Autodesk Inventor part; units mm, degrees
ref_plane "YZ Plane" through (0, 0, 0) normal (1, 0, 0) x (0, 1, 0)
ref_plane "XZ Plane" through (0, 0, 0) normal (0, 1, 0) x (-1, 0, 0)
ref_plane "XY Plane" through (0, 0, 0) normal (0, 0, 1) x (1, 0, 0)
sketch "Sketch1" plane through (0, 0, 0) normal (0, 1, 0) x (-1, 0, 0)
  line L0 (0, 0) -> (85.48, 0)
  line L1 (85.48, 0) -> (85.48, -127.76)
  line L2 (85.48, -127.76) -> (0, -127.76)
  line L3 (0, -127.76) -> (0, 0)
  line L4 (0, 0) -> (7.0711, -7.0711)
  line L5 (0, 0) -> (10, 0) construction
  circle A0 centre (7.0711, -7.0711) radius 4.7625
  dimension "d0" = 85.48
  dimension "d1" = 127.76
  dimension "offsetDiag" = 10
  dimension "d3" = 45
  dimension "d4" = 9.525
extrude "Extrusion1" add sketch "Sketch1" along normal blind 12.7 contours L0 L1 L2 L3 | A0
sketch "Sketch3" plane through (0, 12.7, 0) normal (0, 1, 0) x (1, 0, 0)
  line L0 (0, 0) -> (0, 127.76)
  line L1 (0, 63.88) -> (-72.5, 63.88)
  line L2 (-140, 121.63) -> (-5, 121.63)
  line L3 (-5, 121.63) -> (-5, 6.13)
  line L4 (-5, 6.13) -> (-140, 6.13)
  line L5 (-140, 6.13) -> (-140, 121.63)
  line L6 (-140, 121.63) -> (-5, 6.13) construction
  line L7 (-5, 121.63) -> (-140, 6.13) construction
  dimension "d23" = 72.5
  dimension "d24" = 135
  dimension "d25" = 115.5
extrude "Extrusion2" cut sketch "Sketch3" against normal blind 2.54
sketch "Sketch4" plane through (0, 12.7, 0) normal (0, 1, 0) x (1, 0, 0)
  line L0 (-5, 121.63) -> (-5, 6.13)
  line L1 (5, 67.055) -> (-5, 67.055)
  line L2 (-5, 67.055) -> (-5, 60.705)
  line L3 (-5, 60.705) -> (5, 60.705)
  line L4 (5, 60.705) -> (5, 67.055)
  line L5 (0, 0) -> (0, 127.76)
  line L6 (5, 67.055) -> (-5, 60.705) construction
  line L7 (-5, 67.055) -> (5, 60.705) construction
  point P0 (0, 63.88)
  point P1 (0, 60.705)
  point P2 (0, 67.055)
  dimension "d28" = 6.35
extrude "Extrusion3" cut sketch "Sketch4" against normal blind 2.54 contours L1 L5 L3 L0
sketch "Sketch5" plane through (0, 12.7, 0) normal (0, 1, 0) x (1, 0, 0)
  line L0 (0, 67.055) -> (0, 60.705)
  line L1 (0, 63.88) -> (-67.5, 63.88)
  circle A0 centre (-67.5, 63.88) radius 13.335
  line L2 (-85.48, 0) -> (0, 0)
  line L3 (-70.04, 127.76) -> (-38.29, 127.76)
  line L4 (-38.29, 127.76) -> (-38.29, 0)
  line L5 (-38.29, 0) -> (-70.04, 0)
  line L6 (-70.04, 0) -> (-70.04, 127.76)
  line L7 (-70.04, 127.76) -> (-38.29, 0) construction
  line L8 (-38.29, 127.76) -> (-70.04, 0) construction
  line L9 (-85.48, 121.63) -> (-5, 121.63)
  line L10 (-68.5166, 121.63) -> (-38.29, 121.63)
  line L11 (-38.29, 121.63) -> (-38.29, 127.76)
  line L12 (-38.29, 127.76) -> (-68.5166, 127.76)
  line L13 (-68.5166, 127.76) -> (-68.5166, 121.63)
  line L14 (-5, 6.13) -> (-85.48, 6.13)
  line L15 (-70.04, 0) -> (-38.29, 0)
  line L16 (-38.29, 0) -> (-38.29, 6.13)
  line L17 (-38.29, 6.13) -> (-70.04, 6.13)
  line L18 (-70.04, 6.13) -> (-70.04, 0)
  circle A1 centre (-67.5, 63.88) radius 14.9695
  point P0 (-54.165, 63.88)
  point P1 (-70.04, 6.13)
  point P2 (-38.29, 121.63)
  dimension "d32" = 26.67
  dimension "d31" = 67.5
  dimension "d33" = 31.75
  dimension "d158" = 29.939
sketch "Sketch22" plane through (0, 12.7, 0) normal (0, 1, 0) x (1, 0, 0)
  line L0 (0, 127.76) -> (-85.48, 127.76)
  line L1 (0, 0) -> (0, 127.76)
  line L2 (-85.48, 127.76) -> (0, 127.76)
  line L3 (0, 127.76) -> (0, 121.1763)
  line L4 (0, 121.1763) -> (-85.48, 121.1763)
  line L5 (-85.48, 121.1763) -> (-85.48, 127.76)
  line L6 (0, 0) -> (0, 60.705)
  line L7 (-5, 6.13) -> (-85.48, 6.13)
  line L8 (0, 0) -> (-85.48, 0)
  line L9 (-85.48, 0) -> (-85.48, 6.13)
  line L10 (-85.48, 6.13) -> (0, 6.13)
  line L11 (0, 6.13) -> (0, 0)
extrude "Extrusion16" add sketch "Sketch22" along normal blind 6.35
sketch "Sketch23" plane through (0, 19.05, 0) normal (0, 1, 0) x (1, 0, 0)
  line L0 (0, 127.76) -> (-85.48, 127.76)
  line L1 (-85.48, 0) -> (0, 0)
  line L2 (-85.48, 127.76) -> (0, 127.76)
  line L3 (0, 127.76) -> (0, 0)
  line L4 (0, 0) -> (-85.48, 0)
  line L5 (-85.48, 0) -> (-85.48, 127.76)
extrude "Extrusion17" add sketch "Sketch23" along normal blind 25.4
extrude "Extrusion18" cut sketch "Sketch5" along normal blind 38.1 contours A1 L6 A0 L1 | L1 A0 L6 A1 | A0 L6 | L6 A0 A1 | L6 A0
pattern_linear "Rectangular Pattern2" count 3 spacing 40 along (0, 0, 1) count 2 spacing 40 along (1, 0, 0) of "Extrusion18" first direction both ways yes
sketch "Sketch24" plane through (-85.48, 0, -127.76) normal (-1, 0, 0) x (0, 0, 1)
  line L0 (121.63, 10.16) -> (6.13, 10.16)
  line L1 (63.88, 10.16) -> (63.88, 19.05)
  line L2 (78.8495, 19.05) -> (48.9105, 19.05)
  line L3 (6.13, 8.255) -> (121.63, 8.255)
  line L4 (121.63, 8.255) -> (121.63, 20.955)
  line L5 (121.63, 20.955) -> (6.13, 20.955)
  line L6 (6.13, 20.955) -> (6.13, 8.255)
  line L7 (6.13, 8.255) -> (121.63, 20.955) construction
  line L8 (121.63, 8.255) -> (6.13, 20.955) construction
  point P0 (127.76, 0)
  point P1 (63.88, 14.605)
  dimension "d167" = 12.7
extrude "Extrusion19" cut sketch "Sketch24" against normal up to surface (80.48 mm away)
properties part number "StirredVialHolder"
Read the model definition and answer for the solid it produces. Units are mm, in the model's axes. A direction names the side the tool comes from. Coordinates: 2 decimals unless noted, no trailing zeros. Write each loop counter-clockwise with the first axis right and the second up, starting at its lowest first coordinate (ties: lowest second). Pieces come first, ordered by that corner, then holes. Notation, with made-up numbers: (55.5, -17.75) -> (86.5, -17.75) arc R35 cw to (86.5, 19.25) -> close; hole circle Ø9 at (24, 23). An arc over 180 degrees is marked (long way). Answer as a JSON object with one key per item and string values.
Q1. Flat-ended cylindrical pins translate along their axes: pin 1 Ø4 at (y, z) = (14.5, -52) entering from -X; pin 2 Ø4 at (x, z) = (-35, -111.5) entering from +Y (3 decimals). Find the tip coordinate at first contact, or state that the pin passes through.
The answers:
{"pin 1": "stops at x = -5", "pin 2": "stops at y = 8.255"}
Q2. The part is cut by section A-A on z = -63.88. Give the number of separate pieces and of enclosed holes in the cut face, then the cut area to 3 significant figures.
The answers:
{"separate pieces": "4", "enclosed holes": "0", "area": "1,330 mm2"}
Q3. Consider line 1 (Z direction, x = -67.5, y = 37.5); line 2 (X direction, y = 29, z = -23); line 3 (Y direction, x = -26, z = -120) (3 decimals). Determine where each line is inside the solid, lowest interval first. Write a range as [from, to].
The answers:
{"line 1": "z = [-127.76, -118.85], [-88.91, -78.85], [-48.91, -38.85], [-8.91, 0]", "line 2": "x = [-85.48, -82.44], [-52.56, -42.44], [-12.56, 0]", "line 3": "y = [0, 8.255], [20.955, 44.45]"}
Q4. The part is cut by section D-D on z = -46.5. Give the vertices of the cut face in (x, y) (3 decimals), then the cut area to 3 significant figures.
The answers:
{"outline": "(-85.48, 0) -> (0, 0) -> (0, 12.7) -> (-5, 12.7) -> (-5, 8.255) -> (-85.48, 8.255) -> close; (-85.48, 20.955) -> (-5, 20.955) -> (-5, 19.05) -> (0, 19.05) -> (0, 44.45) -> (-85.48, 44.45) -> close", "area": "2,750 mm2"}
Q5. The part is cut by section C-C on y = 34. Give the vertices of the cut face in (x, z), then the cut area to 3 significant figures.
The answers:
{"outline": "(-85.48, -127.76) -> (0, -127.76) -> (0, 0) -> (-85.48, 0) -> close; hole circle Ø29.94 at (-67.5, -103.88); hole circle Ø29.94 at (-67.5, -63.88); hole circle Ø29.94 at (-67.5, -23.88); hole circle Ø29.94 at (-27.5, -103.88); hole circle Ø29.94 at (-27.5, -63.88); hole circle Ø29.94 at (-27.5, -23.88)", "area": "6,700 mm2"}
Q6. Determine the mould class of faces 5 (the flat face through (-2, 12.7, -33)), 6 (the flat face through (-43, 22, 0)), 7 (the flat face through (0, 22, -65)), 8 (the cylindrical face through (-82.455, 32.538, -63.222)) for opening direction Z: pulls with the +Z half, pulls with the -Z half, needs draft (parallel to the pull), parting line crosses it, or undercut.
The answers:
{"face 5": "undercut", "face 6": "pulls with the +Z half", "face 7": "needs draft", "face 8": "undercut"}
Q7. A tool of negligible diameter and unlimited length cuts with its end or side. For faces 1 (the cylindrical face through (-79.38, 32.54, -112.99)), 2 (the flat face through (-46, 15, -121.63)), 3 (the flat face through (-2, 11, -67.055)), 4 (the flat face through (-42, 22, -127.76)), from which of +Z, -Z, +X, -X, +Y, -Y can it reach the whole face along a straight path? Write none if from no direction.
The answers:
{"face 1": "+Y", "face 2": "-X", "face 3": "+X, -X", "face 4": "-Z, +X, -X, +Y, -Y"}
